Design review of the part built by this model. Coordinates are the model's own, in mm. A direction names the side the tool comes from. Give positions to 0.01 mm unless a question says otherwise; leave off trailing zeros. Order: outer loops, then holes, each group sorted by start corner. A loop starts at its lowest first (then second) coordinate and runs counter-clockwise, first axis right, second up. Notation, with made-up numbers: M 9,49.5 L 52,49.5 A23 cw 52,60.5 Z; hole C -15.5,77.5 d9. An arc over 180 degrees is marked long. Answer as a JSON object with one key per item and string values.
from build123d import *

# Parameters (mm, degrees)
BOSS_EXTRUDE1_DEPTH            = 0.508
CUT_EXTRUDE1_DEPTH             = 1.508
CIRPATTERN1_COUNT              = 5
CIRPATTERN1_ANGLE              = 120
FILLET1_R                      = 1
F_4_CLEARANCE_HOLE1_AT_2_COUNT = 2
F_4_CLEARANCE_HOLE1_AT_2_PITCH = 13
CIRPATTERN2_COUNT              = 4
CIRPATTERN2_ANGLE              = 165
CUT_EXTRUDE2_DEPTH             = 1.508


with BuildPart() as part:
    # Sketch1 → Boss-Extrude1 (new body)
    with BuildSketch(Plane.XY):
        with BuildLine():
            Line((63.498031466, 0.5), (20.758479237, 0.5))
            ThreePointArc((20.758479237, 0.5), (0, 20.7645), (-20.758479237, 0.5))
            Line((-20.758479237, 0.5), (-63.498031466, 0.5))
            ThreePointArc((-63.498031466, 0.5), (0, 63.5), (63.498031466, 0.5))
        make_face()
    extrude(amount=BOSS_EXTRUDE1_DEPTH)

    # Sketch2 → Cut-Extrude1 (cut, through all)
    with BuildSketch(Plane(origin=(0, 0, 0), x_dir=(-1, 0, 0), z_dir=(0, 0, -1))):
        with BuildLine():
            Line((29.810889132, 17.5), (17.856281105, 10.598003837))
            Line((17.856281105, 10.598003837), (18.106281105, 10.164991136))
            Line((18.106281105, 10.164991136), (30.060889132, 17.066987298))
            ThreePointArc((30.060889132, 17.066987298), (30.743901834, 17.75), (29.810889132, 17.5))
        make_face()
    cut_extrude1 = extrude(amount=-CUT_EXTRUDE1_DEPTH, mode=Mode.SUBTRACT)

    # CirPattern1: Cut-Extrude1 ×5 about axis
    cirpattern1_axis = Axis((0, 0, 0), (0, 0, -1))
    for i in range(1, CIRPATTERN1_COUNT):
        add(cut_extrude1.rotate(cirpattern1_axis, i * CIRPATTERN1_ANGLE / (CIRPATTERN1_COUNT - 1)), mode=Mode.SUBTRACT)

    # Fillet1
    fillet1_edges = [part.edges().sort_by_distance(p)[0] for p in [
        (-18.106281105, 10.164991136, 0.254),
        (-17.856281105, 10.598003837, 0.254),
        (-10.598003837, 17.856281105, 0.254),
        (-10.164991136, 18.106281105, 0.254),
        (-0.25, 20.762994973, 0.254),
        (0.25, 20.762994973, 0.254),
        (10.164991136, 18.106281105, 0.254),
        (10.598003837, 17.856281105, 0.254),
        (18.106281105, 10.164991136, 0.254),
        (17.856281105, 10.598003837, 0.254),
        (63.498031466, 0.5, 0.254),
        (20.758479237, 0.5, 0.254),
        (-63.498031466, 0.5, 0.254),
        (-20.758479237, 0.5, 0.254),
    ]]
    fillet(fillet1_edges, radius=FILLET1_R)

    # Sketch3 → #4 Clearance Hole1 (revolve, cut)
    with BuildSketch(Plane(origin=(59.486691682, 7.831571533, 0), x_dir=(0, 1, 0), z_dir=(1, 0, 0))):
        Polygon((0, 0), (0, 136.775187864), (1.4732, 135.89), (1.4732, 0), align=None)
    f_4_clearance_hole1 = revolve(axis=Axis((59.486691682, 7.831571533, -6.35), (0, 0, 1)), mode=Mode.SUBTRACT)

    # #4 Clearance Hole1 at 2: #4 Clearance Hole1 ×2
    with Locations(*[Vector(-0.991444861, -0.130526192, 0) * (i * F_4_CLEARANCE_HOLE1_AT_2_PITCH) for i in range(1, F_4_CLEARANCE_HOLE1_AT_2_COUNT)]):
        add(f_4_clearance_hole1, mode=Mode.SUBTRACT)

    # CirPattern2: #4 Clearance Hole1 ×4 about axis
    cirpattern2_axis = Axis((0, 0, 0), (0, 0, 1))
    for i in range(1, CIRPATTERN2_COUNT):
        add(f_4_clearance_hole1.rotate(cirpattern2_axis, i * CIRPATTERN2_ANGLE / (CIRPATTERN2_COUNT - 1)), mode=Mode.SUBTRACT)

    # CirPattern2 copy 1 sketch → CirPattern2 copy 1 (revolve, cut)
    with BuildSketch(Plane(origin=(21.702184822, 41.689509159, 0), x_dir=(-0.819152044, 0.573576436, 0), z_dir=(0.573576436, 0.819152044, 0))):
        Polygon((0, 0), (0, 136.775187864), (1.4732, 135.89), (1.4732, 0), align=None)
    revolve(axis=Axis((21.702184822, 41.689509159, -6.35), (0, 0, 1)), mode=Mode.SUBTRACT)

    # CirPattern2 copy 2 sketch → CirPattern2 copy 2 (revolve, cut)
    with BuildSketch(Plane(origin=(-21.702184822, 41.689509159, 0), x_dir=(-0.939692621, -0.342020143, 0), z_dir=(-0.342020143, 0.939692621, 0))):
        Polygon((0, 0), (0, 136.775187864), (1.4732, 135.89), (1.4732, 0), align=None)
    revolve(axis=Axis((-21.702184822, 41.689509159, -6.35), (0, 0, 1)), mode=Mode.SUBTRACT)

    # CirPattern2 copy 3 sketch → CirPattern2 copy 3 (revolve, cut)
    with BuildSketch(Plane(origin=(-46.597908485, 6.134731034, 0), x_dir=(-0.258819045, -0.965925826, 0), z_dir=(-0.965925826, 0.258819045, 0))):
        Polygon((0, 0), (0, 136.775187864), (1.4732, 135.89), (1.4732, 0), align=None)
    revolve(axis=Axis((-46.597908485, 6.134731034, -6.35), (0, 0, 1)), mode=Mode.SUBTRACT)

    # Sketch5 → Cut-Extrude2 (cut, through all)
    with BuildSketch(Plane(origin=(0, 0, 0), x_dir=(-1, 0, 0), z_dir=(0, 0, -1))):
        with BuildLine():
            Line((-4.5, 55), (4.5, 55))
            ThreePointArc((4.5, 55), (6.5, 53), (4.5, 51))
            Line((4.5, 51), (-4.5, 51))
            ThreePointArc((-4.5, 51), (-6.5, 53), (-4.5, 55))
        make_face()
    extrude(amount=-CUT_EXTRUDE2_DEPTH, mode=Mode.SUBTRACT)


solid = part.part
(1) To check wall thickness, follow L1, parallel to X at y = 21.5, z = 0.1; L2, parallel to X at y = 22.5, z = 0.1; L3, parallel to Y at x = 23, z = 0.4. State the ranges of each line that lie inside material, in increasing order. Write a range as from..to.
Checked values:
{"L1": "x = -59.75..-12.7, -12.12..-0.28, 0.28..12.12, 12.7..59.75", "L2": "x = -59.38..-13.28, -12.7..-0.25, 0.25..12.7, 13.28..59.38", "L3": "y = 0.5..12.99, 13.57..40.99, 42.39..59.19"}
(2) Draft analysis for pull direction Y (two halves, no side actions). For faces 1 (the flat face through (24.174, 14.245, 0.25)), 2 (the cylindrical face through (-27.9, 54.68, 0.25)), 3 (the cylindrical face through (-1.375, 63.485, 0.25)), 4 (the cylindrical face through (20.04, 5.43, 0.25)), state which applies: +Y half, -Y half, draft (parallel to the pull), parting line (faces both ways), or undercut.
Checked values:
{"face 1": "undercut", "face 2": "undercut", "face 3": "+Y half", "face 4": "-Y half"}
(3) Insertion check: pin 1 (2.5 mm diameter, centred on x = -27.7, y = 53.22, fed in from +Z). The pin has a flat end and moves straight along its axis. Give the tip position at first contact, or say it passes through.
Checked values:
{"pin 1": "passes through"}
(4) We need section A-A (y = 23.5). Write out the cut boundary in (x, z).
Checked values:
{"outline": "M -58.99,0 L -13.86,0 L -13.86,0.51 L -58.99,0.51 Z; M -13.28,0 L -0.25,0 L -0.25,0.51 L -13.28,0.51 Z; M 0.25,0 L 13.28,0 L 13.28,0.51 L 0.25,0.51 Z; M 13.86,0 L 58.99,0 L 58.99,0.51 L 13.86,0.51 Z"}
(5) We need section C-C (x = -54). Write out the cut boundary in (y, z), plus the area to 3 significant figures.
Checked values:
{"outline": "M 0.5,0 L 33.41,0 L 33.41,0.51 L 0.5,0.51 Z", "area": "16.7 mm^2"}
(6) We need section B-B (z = 0.4). Count the separate pieces of the cut face and the enclosed holes in it, plus the area to 3 significant figures.
Checked values:
{"separate pieces": "1", "enclosed holes": "9", "area": "5,470 mm^2"}
(7) Tool access review of faces 5 (the cylindrical face through (-5.32, 20.07, 0.25)), 6 (the flat face through (14.335, 24.33, 0.25)), 7 (the flat face through (1, 25, 0.508)): name each direction out of +Z, -Z, +X, -X, +Y, -Y from which nothing blocks a thin tool from reaching the whole face with its end or side.
Checked values:
{"face 5": "+Z, -Z, -Y", "face 6": "+Z, -Z", "face 7": "+Z, +X, -X, +Y, -Y"}
